from build123d import *

# Parameters (mm, degrees)
F0_R     = 6.1595
F1_DEPTH = 25.4
F3_DEPTH = 6.35
F4_R     = 6.1595
F5_DEPTH = 31.75
F6_R     = 4.441025895
F7_DEPTH = 44.45
F8_R     = 4.445
F9_DEPTH = 29.21


with BuildPart() as f1:
    # F0 (on Front) → F1 (new body)
    with BuildSketch(Plane.XZ):
        with Locations((10.16, 0)):
            Circle(F0_R)
    extrude(amount=F1_DEPTH)



with BuildPart() as f1b:
    # F0 (on Front) → F1, piece 2 (new body)
    with BuildSketch(Plane.XZ):
        with Locations((-10.16, 0)):
            Circle(F0_R)
    extrude(amount=F1_DEPTH)


with BuildPart() as f1_1:
    add(f1.part)

    add(f1b.part)  # F3 merges F1b
    # F2 (on Front) → F3 (join, symmetric)
    with BuildSketch(Plane.XZ):
        with BuildLine():
            ThreePointArc((-8.89, 8.89), (-17.78, 0), (-8.89, -8.89))
            Line((-8.89, -8.89), (8.89, -8.89))
            ThreePointArc((8.89, -8.89), (17.78, 0), (8.89, 8.89))
            Line((8.89, 8.89), (-8.89, 8.89))
        make_face()
    extrude(amount=F3_DEPTH, both=True)

    # F4 (on Right) → F5 (join)
    with BuildSketch(Plane.YZ):
        Circle(F4_R)
    extrude(amount=F5_DEPTH)

    # F6 (on face) → F7 (cut)
    with BuildSketch(Plane.YZ.offset(31.75)):
        Circle(F6_R)
    extrude(amount=-F7_DEPTH, mode=Mode.SUBTRACT)

    # F8 (on face) → F9 (cut)
    with BuildSketch(Plane.XZ.offset(25.4)):
        with Locations((-10.16, 0)):
            Circle(F8_R)
        with Locations((10.16, 0)):
            Circle(F8_R)
    extrude(amount=-F9_DEPTH, mode=Mode.SUBTRACT)


solid = f1_1.part
Model file for the job. Use its own axes, mm. A direction names the side the tool comes from. Round coordinates to 2 decimals unless told otherwise and drop trailing zeros. Order: outer loops, then holes, each group sorted by start corner. A loop starts at its lowest first (then second) coordinate and runs counter-clockwise, first axis right, second up.
(1) Pull direction X, two halves, no side cores. Call faces 4 (the face through (-14.6, -11, 0.2)), 5 (the face through (-17.778, -0.089, 0.195)), 6 (the face through (31.75, 4, -3)), 7 (the face through (0, 6.35, 0)): released by +X, released by -X, zero draft, split by the parting line, or undercut.
(2) Band-saw the part on A-A (z = 0). Give the number of separate pieces and of enclosed holes in the cut face, then the cut area to 3 significant figures.
(3) Band-saw the part on D-D (y = -5). List the corners of the cut face in (x, z) (3 decimals).
(4) Band-saw the part on B-B (y = -10.5). List the corners of the cut face in (x, z) (1 decimal), then the cut area to 3 significant figures.
(5) Drill centre lines: line 1 (Y direction, x = 2.5, z = 0); line 2 (Z direction, x = 10, y = -19); line 3 (X direction, y = -24, z = -2). Where is each one in solid material? Low to high.
(6) 3-axis set-ups, long thin cutter, end or side, ignore diameter. For faces 1 (the face through (0, 0, -8.89)), 2 (the face through (-7.318, -15.742, -5.465)), 3 (the face through (-11.77, -0.04, -4.44)): which of +Z, -Z, +X, -X, +Y, -Y reach the whole face in a straight line?
(7) Pin check, flat tips, straight feed: pin 1 (1 mm diameter, centred on y = -20, z = -2.5, fed in from +X); pin 2 (9 mm diameter, centred on x = -11, z = -0.5, fed in from -Y); pin 3 (10 mm diameter, centred on x = 19.5, y = -5, fed in from -Z); pin 4 (5 mm diameter, centred on x = 25.5, z = -7, fed in from -Y). Stop position of each tip, or through.
(8) Band-saw the part on C-C (x = 24.5). List the corners of the cut face in (y, z).
Verdict:
1. face 4: undercut
1. face 5: released by -X
1. face 6: released by +X
1. face 7: zero draft
2. separate pieces: 3
2. enclosed holes: 0
2. area: 310 mm2
3. outline: (-8.89, -8.89) - (8.89, -8.89) arc R8.89 ccw to (17.02, -3.597) - (31.75, -3.597) - (31.75, 3.597) - (17.02, 3.597) arc R8.89 ccw to (8.89, 8.89) - (-8.89, 8.89) arc R8.89 ccw to start; hole circle Ø8.89 at (-10.16, 0); hole circle Ø8.89 at (10.16, 0)
4. outline: circle Ø12.3 at (-10.2, 0); circle Ø12.3 at (10.2, 0); hole circle Ø8.9 at (-10.2, 0); hole circle Ø8.9 at (10.2, 0)
4. area: 114 mm2
5. line 1: y = -6.35 to -4.44, 4.44 to 6.35
5. line 2: z = -6.16 to -4.44, 4.44 to 6.16
5. line 3: x = -15.99 to -14.13, -6.19 to -4.33, 4.33 to 6.19, 14.13 to 15.99
6. face 1: -Z, +X, -X, +Y, -Y
6. face 2: -Y
6. face 3: +X
7. pin 1: stops at x = 15.99
7. pin 2: stops at y = -25.4
7. pin 3: stops at z = -6.9
7. pin 4: stops at y = -4.21
8. outline: circle Ø12.32 at (0, 0); hole circle Ø8.88 at (0, 0)
